Autodesk Inventor part; units mm, degrees
ref_plane "РабПлоскость1" through (-34.9448, 28.465, -130.3508) normal (0, 0, 1) x (1, 0, 0)
ref_plane "YZ Plane" through (0, 0, 0) normal (1, 0, 0) x (0, 1, 0)
ref_plane "XZ Plane" through (0, 0, 0) normal (0, 1, 0) x (-1, 0, 0)
ref_plane "РабПлоскость1" through (-34.9448, 28.465, -130.3508) normal (0, 0, 1) x (1, 0, 0)
ref_plane "РабПлоскость2" through (-162.802, 331.465, 111.3492) normal (0, 0, 1) x (1, 0, 0)
sketch "Эскиз1" plane through (-34.9448, 28.465, -130.3508) normal (0, 0, 1) x (1, 0, 0)
  line L0 (0, 3.6904) -> (-12.8571, 3.6904) construction
  line L1 (0, 3.6904) -> (0, 9.6905)
  line L2 (-12.8571, 9.6905) -> (0, 9.6905)
  line L3 (-12.8571, 3.6904) -> (-12.8571, 9.6905)
  line L4 (25.7143, 3.6904) -> (12.8571, 3.6904) construction
  line L5 (25.7143, 3.6904) -> (25.7143, 9.6905)
  line L6 (12.8571, 9.6905) -> (25.7143, 9.6905)
  line L7 (12.8571, 3.6904) -> (12.8571, 9.6905)
  line L8 (51.4286, 3.6904) -> (38.5714, 3.6904) construction
  line L9 (51.4286, 3.6904) -> (51.4286, 9.6905)
  line L10 (38.5714, 9.6905) -> (51.4286, 9.6905)
  line L11 (38.5714, 3.6904) -> (38.5714, 9.6905)
  line L12 (77.1429, 3.6904) -> (64.2857, 3.6904) construction
  line L13 (77.1429, 3.6904) -> (77.1429, 9.6905)
  line L14 (64.2857, 9.6905) -> (77.1429, 9.6905)
  line L15 (64.2857, 3.6904) -> (64.2857, 9.6905)
  line L16 (0, 3.6904) -> (12.8571, 3.6904)
  line L17 (25.7143, 3.6904) -> (38.5714, 3.6904)
  line L18 (51.4286, 3.6904) -> (64.2857, 3.6904)
  line L19 (-12.8571, 3.6904) -> (-12.8571, -50.3096)
  line L20 (-9.8571, -53.3096) -> (-4.7353, -53.3096)
  line L21 (77.1429, 3.6904) -> (77.1429, -50.3096)
  line L22 (74.1429, -53.3096) -> (69.021, -53.3096)
  line L23 (-1.8571, -53.3096) -> (66.1429, -53.3096) construction
  arc A0 (-1.7452, -56.0663) -> (66.0309, -56.0663) centre (32.1429, -53.3096) ccw
  arc A1 (-1.7452, -56.0663) -> (-4.7353, -53.3096) centre (-4.7353, -56.3096) ccw
  arc A2 (69.021, -53.3096) -> (66.0309, -56.0663) centre (69.021, -56.3096) ccw
  arc A3 (74.1429, -53.3096) -> (77.1429, -50.3096) centre (74.1429, -50.3096) ccw
  arc A4 (-12.8571, -50.3096) -> (-9.8571, -53.3096) centre (-9.8571, -50.3096) ccw
  circle A5 centre (32.1429, -53.3095) radius 2.375
  point P0 (34.9448, -28.465)
  point P1 (77.1429, -53.3096)
  dimension "d0" = 57
  dimension "d1" = 34
  dimension "d2" = 3
  dimension "d3" = 6
  dimension "d14" = 4.75
extrude "Выдавливание1" add sketch "Эскиз1" along normal blind 6
sketch "Эскиз2" plane through (-34.9448, 28.465, -130.3508) normal (0, 0, -1) x (-1, 0, 0)
  line L0 (-4.9286, 3.6904) -> (-4.9286, -2.6596)
  line L1 (-4.9286, -2.6596) -> (-3.6786, -2.6596)
  line L2 (-3.6786, -2.6596) -> (-3.6786, -4.9596)
  line L3 (-3.6786, -4.9596) -> (-4.9286, -4.9596)
  line L4 (-4.9286, -4.9596) -> (-4.9286, -11.3096)
  line L5 (-4.9286, -11.3096) -> (-7.9286, -11.3096)
  line L6 (-7.9286, -11.3096) -> (-7.9286, -4.9596)
  line L7 (-7.9286, -4.9596) -> (-9.1786, -4.9596)
  line L8 (-9.1786, -4.9596) -> (-9.1786, -2.6596)
  line L9 (-9.1786, -2.6596) -> (-7.9286, -2.6596)
  line L10 (-7.9286, -2.6596) -> (-7.9286, 3.6904)
  line L11 (-56.3571, 3.6904) -> (-59.3571, 3.6904)
  line L12 (-56.3571, 3.6904) -> (-56.3571, -2.6596)
  line L13 (-56.3571, -2.6596) -> (-55.1071, -2.6596)
  line L14 (-55.1071, -2.6596) -> (-55.1071, -4.9596)
  line L15 (-55.1071, -4.9596) -> (-56.3571, -4.9596)
  line L16 (-56.3571, -4.9596) -> (-56.3571, -11.3096)
  line L17 (-56.3571, -11.3096) -> (-59.3571, -11.3096)
  line L18 (-59.3571, -11.3096) -> (-59.3571, -4.9596)
  line L19 (-59.3571, -4.9596) -> (-60.6071, -4.9596)
  line L20 (-60.6071, -4.9596) -> (-60.6071, -2.6596)
  line L21 (-60.6071, -2.6596) -> (-59.3571, -2.6596)
  line L22 (-59.3571, -2.6596) -> (-59.3571, 3.6904)
  line L23 (-56.3571, 3.6904) -> (-59.3571, 3.6904)
  line L24 (-4.9286, 3.6904) -> (-7.9286, 3.6904)
  point P0 (-34.9448, -28.465)
  point P1 (-6.4286, 0)
  dimension "d9" = 5.5
  dimension "d10" = 2.3
  dimension "d11" = 15
extrude "Выдавливание2" cut sketch "Эскиз2" against normal blind 6
sketch "Эскиз4" plane through (29.3409, 38.1554, -130.3508) normal (0, 1, 0) x (1, 0, 0)
  line L0 (-77.1429, 0) -> (-77.1429, -6)
  line L1 (12.8571, 0) -> (-77.1429, 0)
  line L2 (-77.1429, 0) -> (-77.1429, -6)
  line L3 (-77.1429, -6) -> (12.8571, -6)
  line L4 (12.8571, -6) -> (12.8571, 0)
  point P0 (-29.3409, -130.3508)
extrude "Выдавливание3" cut sketch "Эскиз4" against normal blind 1
equation "\"d4\" = d3"
equation "\"d12\" = d3"
properties part number "wheel1"
Design review of the part built by this model. Coordinates are the model's own, in mm. A direction names the side the tool comes from. Give positions to 0.01 mm unless a question says otherwise; leave off trailing zeros. Loops run counter-clockwise (first coordinate to the right, second up) from the corner with the lowest first, then second, coordinate; pieces in that order, holes last. Notation, with made-up numbers: (-35.5, 65.25) -> (-14.5, 65.25) arc R21 cw to (-14.5, 70.25) -> close; hole circle Ø8 at (-1, -0.5). An arc over 180 degrees is marked (long way). One line per question, with ' | ' between items. Start each with the question number.
(1) We need section A-A (x = -7). State the section outline as (y, z) points, and give its area (3 significant figures).
(2) For line 1 (X direction, y = 24, z = -129.65); line 2 (X direction, y = 32.5, z = -125.45); line 3 (X direction, y = 17.5, z = -126.6), list the stretches that pass through material, from the lowest coordinate up.
(3) We need section B-B (y = -43). State the section outline as (x, z) points, and give its area (3 significant figures).
(4) Insertion check: P1, Ø1.5, axis at x = 36, z = -127, coming from the -Y side; P2, Ø2.5, axis at x = 26.5, z = -127.5, coming from the +Y side; P3, Ø1, axis at x = -23.5, z = -129, coming from the -Y side. Each pin has a flat end and moves straight along its axis. Give the tip position at first contact, or say it passes through.
(5) For faces 1 (the face through (-31.266, 25, -127)), 2 (the face through (21.412, 20, -127)), 3 (the face through (36, 37.155, -127)), list the 3-axis set-ups (+Z, -Z, +X, -X, +Y, -Y) from which the entire face can be reached by the end or side of a thin tool; tool diameter is ignored.
(6) Draft analysis for pull direction Y (two halves, no side actions). For faces 4 (the face through (20.162, 25, -127)), 5 (the face through (-41, 37.155, -127)), 6 (the face through (-27.016, 20, -127)), 7 (the face through (32.02, -25.66, -127.39)), state which applies: +Y half, -Y half, draft (parallel to the pull), parting line (faces both ways), or undercut.
The answers:
1) outline: (-58.58, -130.35) -> (32.16, -130.35) -> (32.16, -124.35) -> (-58.58, -124.35) -> close | area: 544 mm^2
2) line 1: x = -47.8 to -31.27, -25.77 to 20.16, 25.66 to 42.2 | line 2: x = -47.8 to -34.94, -22.09 to -9.23, 3.63 to 16.48, 29.34 to 42.2 | line 3: x = -47.8 to -30.02, -27.02 to 21.41, 24.41 to 42.2
3) outline: (-31.55, -130.35) -> (25.94, -130.35) -> (25.94, -124.35) -> (-31.55, -124.35) -> close | area: 345 mm^2
4) P1: stops at y = -24.84 | P2: stops at y = 32.16 | P3: stops at y = -52.19
5) face 1: +Z, -Z | face 2: +Z, -Z, +Y | face 3: +Z, -Z, +X, -X, +Y
6) face 4: undercut | face 5: +Y half | face 6: draft | face 7: -Y half
